The listing builds one solid part. Answer for the finished solid, in the listing's coordinates (mm). A direction names the side the tool comes from. Coordinates: 2 decimals unless noted, no trailing zeros. Order: outer loops, then holes, each group sorted by start corner. A loop starts at its lowest first (then second) coordinate and runs counter-clockwise, first axis right, second up.
from build123d import *

# Parameters (mm, degrees)
SKETCH_1_R          = 3.5
EXTRUDE_1_DEPTH     = 3.9
SKETCH_2_R          = 2
EXTRUDE_2_DEPTH     = 10
CUT_EXTRUDE_1_DEPTH = 2.4


with BuildPart() as part:
    # 草图1 → 凸台-拉伸1 (new body)
    with BuildSketch(Plane(origin=(0, 0, 0), x_dir=(1, 0, 0), z_dir=(0, 1, 0))):
        Circle(SKETCH_1_R)
    extrude(amount=EXTRUDE_1_DEPTH)

    # 草图2 → 凸台-拉伸2 (add)
    with BuildSketch(Plane(origin=(0, 3.9, 0), x_dir=(1, 0, 0), z_dir=(0, 1, 0))):
        Circle(SKETCH_2_R)
    extrude(amount=EXTRUDE_2_DEPTH)

    # 草图3 → 切除-拉伸1 (cut)
    with BuildSketch(Plane.XZ):
        Polygon((1.725, 0), (0.8625, 1.493893822), (-0.8625, 1.493893822), (-1.725, 0), (-0.8625, -1.493893822), (0.8625, -1.493893822), align=None)
    extrude(amount=-CUT_EXTRUDE_1_DEPTH, mode=Mode.SUBTRACT)


solid = part.part
1) A tool of negligible diameter and unlimited length cuts with its end or side. For faces 4 (the face through (2, 3.9, 2)), 5 (the face through (3.233, 1.923, 1.341)), 6 (the face through (0, 1, -1.494)), from which of +Z, -Z, +X, -X, +Y, -Y can it reach the whole face along a straight path? Write none if from no direction.
2) Consider L1, parallel to Y at x = 2.25, z = -2.25; L2, parallel to X at y = 9.25, z = 0; L3, parallel to Y at x = -0.75, z = -0.5. Determine where each line is inside the solid, lowest interval first.
3) Each of these flat-tipped pins is pushed along its axis until it touches: P1, Ø1, axis at y = 2.5, z = -2, coming from the -X side; P2, Ø1.5, axis at x = -1, z = 3, coming from the +Y side; P3, Ø4, axis at x = 0.5, y = 11.5, coming from the +Z side. Where does it stop, or does it pass through?
4) Section C-C (y = 7.5) is taken. Give the vertices of the cut face in (x, z).
5) Section A-A (x = 0) is taken. Give the vertices of the cut face in (y, z).
6) Determine the mould class of faces 1 (the face through (0, 9, 2)), 2 (the face through (0, 0, 2)), 3 (the face through (1.3, 1.18, 0.74)) for opening direction X: released by +X, released by -X, zero draft, split by the parting line, or undercut.
7) Section B-B (z = 1) is taken. Give the vertices of the cut face in (x, y).
8) Section D-D (z = -1.75) is taken. Give the vertices of the cut face in (x, y), then the cut area to 3 significant figures.
Filled sheet:
1. face 4: +Y
1. face 5: +Y, -Y
1. face 6: -Y
2. L1: y = 0 to 3.9
2. L2: x = -2 to 2
2. L3: y = 2.4 to 13.9
3. P1: stops at x = -3.16
3. P2: stops at y = 3.9
3. P3: stops at z = 2
4. outline: circle Ø4 at (0, 0)
5. outline: (0, -3.5) - (3.9, -3.5) - (3.9, -2) - (13.9, -2) - (13.9, 2) - (3.9, 2) - (3.9, 3.5) - (0, 3.5) - (0, 1.49) - (2.4, 1.49) - (2.4, -1.49) - (0, -1.49) - close
6. face 1: split by the parting line
6. face 2: zero draft
6. face 3: undercut
7. outline: (-3.35, 0) - (-1.15, 0) - (-1.15, 2.4) - (1.15, 2.4) - (1.15, 0) - (3.35, 0) - (3.35, 3.9) - (1.73, 3.9) - (1.73, 13.9) - (-1.73, 13.9) - (-1.73, 3.9) - (-3.35, 3.9) - close
8. outline: (-3.03, 0) - (3.03, 0) - (3.03, 3.9) - (0.97, 3.9) - (0.97, 13.9) - (-0.97, 13.9) - (-0.97, 3.9) - (-3.03, 3.9) - close
8. area: 43.0 mm2
